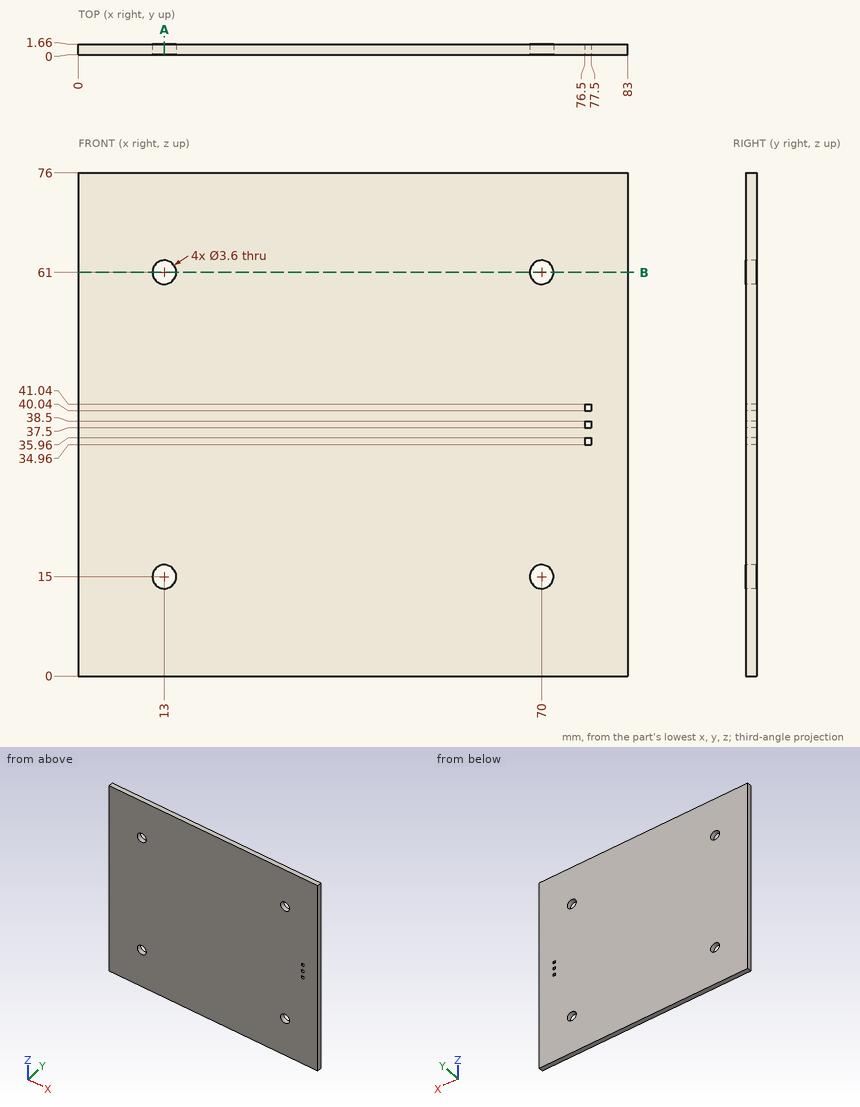
Design review of the part shown in the three views and the two pictorial views. Dimensions are in mm from the part's minimum x, y and z. Round coordinates to 2 decimals unless told otherwise and drop trailing zeros. Write each loop counter-clockwise with the first axis right and the second up, starting at its lowest first coordinate (ties: lowest second). Pieces come first, ordered by that corner, then holes. Notation, with made-up numbers: M 48,50 L 85,50 A24 ccw 85,61 Z; hole C 48,79.5 d7. An arc over 180 degrees is marked long. One line per item, written item: value. Start each with the question number.
1. To check wall thickness, follow probe 1 along Z at (x, y) = (70, 0.7); probe 2 along X at (y, z) = (0.3, 61). State the ranges of each line that lie inside material, in increasing order. Write a range as from..to.
2. Take a section at B-B on z = 61. State the section outline as (x, y) points, then the cut area to 3 significant figures.
3. Clearance check with flat-ended pins moving along their axes: P1, Ø6, axis at x = 13, z = 15, coming from the +Y side; P2, Ø2, axis at x = 70, z = 15, coming from the +Y side. State where each tip first meets the part, or that it passes through.
4. Take a section at A-A on x = 13. State the section outline as (y, z) points, then the cut area to 3 significant figures.
Computed:
1. probe 1: z = 0..13.2, 16.8..59.2, 62.8..76
1. probe 2: x = 0..11.2, 14.8..68.2, 71.8..83
2. outline: M 0,0 L 11.2,0 L 11.2,1.66 L 0,1.66 Z; M 14.8,0 L 68.2,0 L 68.2,1.66 L 14.8,1.66 Z; M 71.8,0 L 83,0 L 83,1.66 L 71.8,1.66 Z
2. area: 126 mm²
3. P1: stops at y = 1.66
3. P2: passes through
4. outline: M 0,0 L 1.66,0 L 1.66,13.2 L 0,13.2 Z; M 0,16.8 L 1.66,16.8 L 1.66,59.2 L 0,59.2 Z; M 0,62.8 L 1.66,62.8 L 1.66,76 L 0,76 Z
4. area: 114 mm²
